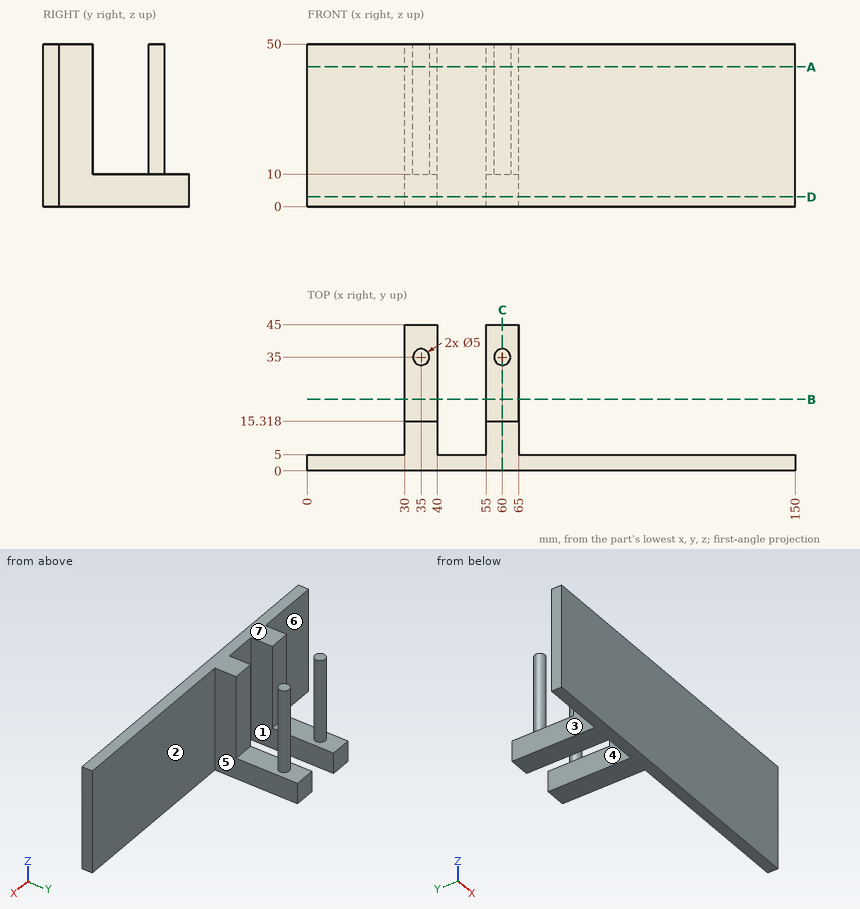
Can you work these out from the drawing? Everything is in mm from the part's minimum corner. A direction names the side the tool comes from. Coordinates: 2 decimals unless noted, no trailing zeros. Loops run counter-clockwise (first coordinate to the right, second up) from the corner with the lowest first, then second, coordinate; pieces in that order, holes last. Notation, with made-up numbers: M -39.5,54 L -18.5,54 A21 cw -18.5,70 Z; hole C -7,-28.75 d11. An arc over 180 degrees is marked long. Put each result on its own line as item: value. Start each with the question number.
(1) Will these pins go through, and if not, where does the flat tip stop? P1, Ø5, axis at x = 60.5, z = 38, coming from the +Y side; P2, Ø10, axis at y = 39, z = 15.5, coming from the -X side; P3, Ø5, axis at x = 59, y = 24.5, coming from the +Z side.
(2) I need wall thicknesses on line 1 (X direction, y = 26.5, z = 5.5); line 2 (Y direction, x = 19.5, z = 35); line 3 (Z direction, x = 58, y = 21.5). Which ranges of each line are inside material? Lowest first, please. Write a range as from..to.
(3) Suppose I cut it at D-D on z = 3. Please give me the cut outline in (x, y).
(4) For the marked faces 5, 6 and 7, which set-ups out of +Z, -Z, +X, -X, +Y, -Y let a thin tool reach every point of the face, with its end or its side?
(5) Thinking about a two-plate mould opening in X: for the marked faces 1, 2, 3 and 4, which applies, pulls with the +X half, pulls with the -X half, needs draft (parallel to the pull), parting line crosses it, or undercut?
(6) Suppose I cut it at B-B on y = 22. Please give me the cut outline in (x, z), then the cut area to 3 significant figures.
(7) Suppose I cut it at C-C on x = 60. Please give me the cut outline in (y, z), then the cut area to 3 significant figures.
(8) Suppose I cut it at A-A on z = 43. Please give me the cut outline in (x, y).
Solutions:
1. P1: stops at y = 37.5
1. P2: stops at x = 32.5
1. P3: stops at z = 10
2. line 1: x = 30..40, 55..65
2. line 2: y = 0..5
2. line 3: z = 0..10
3. outline: M 0,0 L 150,0 L 150,5 L 65,5 L 65,45 L 55,45 L 55,5 L 40,5 L 40,45 L 30,45 L 30,5 L 0,5 Z
4. face 5: +Z, -Z, +X, +Y
4. face 6: +Z, -Z, -X, +Y
4. face 7: +Z, +X, -X, +Y, -Y
5. face 1: undercut
5. face 2: needs draft
5. face 3: pulls with the -X half
5. face 4: undercut
6. outline: M 30,0 L 40,0 L 40,10 L 30,10 Z; M 55,0 L 65,0 L 65,10 L 55,10 Z
6. area: 200 mm2
7. outline: M 0,0 L 45,0 L 45,10 L 37.5,10 L 37.5,50 L 32.5,50 L 32.5,10 L 15.32,10 L 15.32,50 L 0,50 Z
7. area: 1,260 mm2
8. outline: M 0,0 L 150,0 L 150,5 L 65,5 L 65,15.32 L 55,15.32 L 55,5 L 40,5 L 40,15.32 L 30,15.32 L 30,5 L 0,5 Z; C 35,35 d5; C 60,35 d5
